Input: part model. Units: mm. Frame: model coordinates. A direction names the side the tool comes from. Coordinates: 2 decimals unless noted, no trailing zeros. Loops run counter-clockwise (first coordinate to the right, second up) from the corner with the lowest first, then second, coordinate; pieces in that order, holes last. Notation, with made-up numbers: (-36, 48.5) - (-13, 48.5) arc R24 cw to (-13, 85.5) - close; hole circle Ø2 at (-21, 56). An arc over 180 degrees is marked (long way). Use one line per item in the form item = value.
Autodesk Inventor part; units mm, degrees
ref_plane "YZ Plane" through (0, 0, 0) normal (1, 0, 0) x (0, 1, 0)
ref_plane "XZ Plane" through (0, 0, 0) normal (0, 1, 0) x (-1, 0, 0)
ref_plane "XY Plane" through (0, 0, 0) normal (0, 0, 1) x (1, 0, 0)
sketch "草图1" plane through (0, 0, 0) normal (0, 0, 1) x (1, 0, 0)
  line L0 (598.9577, 75) -> (600, -74.9964)
  line L1 (-601.0423, 75.1267) -> (600, -74.9964) construction
  line L2 (598.9577, 75) -> (-593.8092, -74.3553) construction
  line L3 (-300, 0) -> (-300, 100)
  line L4 (-300, -100) -> (600, -74.9964)
  line L5 (-300, 100) -> (598.9577, 75)
  line L6 (-300, 0) -> (-300, -100)
  line L7 (599.4789, 0) -> (-300, 0)
  line L8 (0, 0) -> (0, -189.9048)
  dimension "d0" = 150
  dimension "d31" = 75
  dimension "d32" = 0
  dimension "d33" = 100
  dimension "d34" = 100
  dimension "d35" = 100
  dimension "d51" = 300
extrude "拉伸1" add sketch "草图1" along normal mid plane 100
sketch "草图2" plane through (0, 0, 0) normal (0, 0, 1) x (1, 0, 0)
  circle A0 centre (-50, -120) radius 15
  line L0 (0, 0) -> (0, -405.8359)
  line L1 (0, 0) -> (-641.787, 0)
  line L2 (-80, -120) -> (-80, -93.888)
  line L3 (-300, -100) -> (600, -74.9964)
  line L4 (-20, -92.2211) -> (-20, -120)
  arc A1 (-80, -120) -> (-20, -120) centre (-50, -120) ccw
  dimension "d8" = 30
  dimension "d9" = 120
  dimension "d10" = 50
  dimension "d28" = 30
extrude "拉伸2" add sketch "草图2" along normal mid plane 100
fillet "圆角1" radius 30 1 edges at (-300, -100, 0)
sketch "草图4" plane through (0, 0, 50) normal (0, 0, 1) x (1, 0, 0)
  arc A0 (-300, -69.155) -> (-269.1669, -99.1434) centre (-270, -69.155) ccw
  circle A1 centre (-270, -69.155) radius 15
  point P0 (0, 0)
  dimension "d15" = 30
extrude "拉伸3" cut sketch "草图4" against normal blind 100
sketch "草图5" plane through (0, 0, 50) normal (0, 0, 1) x (1, 0, 0)
  arc A0 (-300, -69.155) -> (-269.1669, -99.1434) centre (-270, -69.155) ccw
  line L0 (-300, -69.155) -> (-300, 100)
  line L1 (598.9577, 75) -> (-300, 100)
  line L2 (-300, 100) -> (-300, -69.155)
  line L3 (-300, 100) -> (-300, 100)
  line L4 (-300, -69.155) -> (-295.2994, 99.8693)
  line L5 (-295.2994, 99.8693) -> (-300, 100)
  line L6 (598.9577, 75) -> (594.7823, -75.1413)
  line L7 (600, -74.9964) -> (-269.1669, -99.1434)
  line L8 (598.9577, 75) -> (600, -74.9964)
  line L9 (600, -74.9964) -> (598.9577, 75)
  point P0 (0, 0)
  point P1 (-603.2218, 0)
  point P2 (599.4789, 0)
  dimension "d20" = 90
extrude "拉伸4" cut sketch "草图5" against normal blind 100 contours L0 L1 L4 | L6 L8 L7
sketch "草图6" plane through (594.7823, -75.1413, 50) normal (0.9996135, -0.0277992, 0) x (0, 0, -1)
  line L0 (0, 0) -> (0, 150.1994)
  line L1 (0, 150.1994) -> (100, 150.1994)
  line L2 (50, 150.1994) -> (50, 0)
  line L3 (100, 0) -> (0, 0)
  line L4 (100, 150.1994) -> (100, 0)
  line L5 (15, 151) -> (85, 151)
  line L6 (85, 151) -> (85, 20)
  line L7 (85, 20) -> (15, 20)
  line L8 (15, 20) -> (15, 151)
  line L9 (15, 151) -> (85, 20) construction
  line L10 (85, 151) -> (15, 20) construction
  point P0 (50, 58.5778)
  point P1 (50, 85.5)
  point P2 (0, 100.4456)
  point P3 (0, 175.4618)
  point P4 (100, 175.4618)
  point P5 (100, 100.4456)
  dimension "d21" = 70
  dimension "d22" = 131
  dimension "d63" = 20
extrude "拉伸5" cut sketch "草图6" against normal through all contours L8 L5 L6 L1 | L1 L2 L7 L8 | L2 L1 L6 L7
sketch "草图7" plane through (0, 0, 0) normal (0, 0, 1) x (1, 0, 0)
  arc A0 (-300, -69.155) -> (-269.1669, -99.1434) centre (-270, -69.155) ccw
  circle A1 centre (-270, -69.155) radius 42.5
  point P0 (0, 0)
  dimension "d25" = 85
extrude "拉伸6" cut sketch "草图7" along normal mid plane 35
sketch "草图8" plane through (0, 0, 0) normal (0, 0, 1) x (1, 0, 0)
  line L0 (-632.149, 69.2216) -> (221.7891, 45.4736)
  line L1 (-295.2994, 99.8693) -> (-298.9189, -30.2798)
  line L2 (598.9577, 75) -> (-295.2994, 99.8693)
  circle A0 centre (-246.4307, 58.4948) radius 15
  arc A1 (-276.4191, 59.3288) -> (-216.4423, 57.6608) centre (-246.4307, 58.4948) ccw
  line L3 (-276.4191, 59.3288) -> (-275.3072, 99.3133)
  line L4 (-275.3072, 99.3133) -> (-520.3529, 106.128)
  line L5 (-275.3127, 99.114) -> (-215.3359, 97.446)
  line L6 (598.9522, 74.8007) -> (-295.305, 99.67)
  line L7 (-215.3359, 97.446) -> (-216.4423, 57.6608)
  point P0 (0, 0)
  dimension "d36" = 40
  dimension "d37" = 30
  dimension "d38" = 60
  dimension "d39" = 50
  dimension "d40" = 90
  dimension "d41" = 60
extrude "拉伸7" add sketch "草图8" along normal mid plane 70 contours L3 L5 L7 L0 A0 | L0 A0 A1 | A0 L0 | L0 A0
sketch "草图9" plane through (0, 0, 50) normal (0, 0, 1) x (1, 0, 0)
  arc A0 (-276.4191, 59.3288) -> (-216.4423, 57.6608) centre (-246.4307, 58.4948) ccw
  circle A1 centre (-246.4307, 58.4948) radius 15
  point P0 (0, 0)
  dimension "d44" = 30
extrude "拉伸8" cut sketch "草图9" against normal through all
sketch "草图10" plane through (-276.4191, 59.3288, -35) normal (-0.9996135, 0.0277992, 0) x (0, 0, 1)
  line L0 (0, 39.8006) -> (70, 39.8006)
  line L1 (35, 39.8006) -> (35, -30)
  line L2 (0, -30) -> (70, -30)
  line L3 (17.5, 39.8006) -> (52.5, 39.8006)
  line L4 (52.5, 39.8006) -> (52.5, -30)
  line L5 (52.5, -30) -> (17.5, -30)
  line L6 (17.5, -30) -> (17.5, 39.8006)
  line L7 (17.5, 39.8006) -> (52.5, -30) construction
  line L8 (52.5, 39.8006) -> (17.5, -30) construction
  point P0 (35, -51.6216)
  point P1 (35, 4.9003)
  dimension "d47" = 35
extrude "拉伸9" cut sketch "草图10" against normal blind 60
sketch "草图13" plane through (-295.2994, 99.8693, 50) normal (0.0277992, 0.9996135, 0) x (0.9996135, -0.0277992, 0)
  line L0 (0, 15) -> (0, 85)
  line L1 (0, 50) -> (323.6348, 50)
  line L2 (0, 100) -> (31.6549, 100)
  line L3 (200, 0) -> (0, 0)
  line L4 (0, 0) -> (0, 100)
  line L5 (0, 100) -> (200, 100)
  line L6 (200, 100) -> (200, 0)
  line L7 (200, 0) -> (0, 100) construction
  line L8 (0, 0) -> (200, 100) construction
  line L9 (894.6029, 100) -> (894.6029, 0)
  line L10 (844.6029, 100) -> (894.6029, 100)
  line L11 (894.6029, 100) -> (894.6029, 0)
  line L12 (894.6029, 0) -> (844.6029, 0)
  line L13 (844.6029, 0) -> (844.6029, 100)
  line L14 (844.6029, 100) -> (894.6029, 0) construction
  line L15 (894.6029, 100) -> (844.6029, 0) construction
  point P0 (297.9616, 50)
  point P1 (100, 50)
  point P2 (869.6029, 50)
  dimension "d64" = 200
  dimension "d65" = 50
extrude "拉伸12" add sketch "草图13" along normal blind 10
properties part number "DipperParent" material "钢，高强度，低合金"
Q1. First-contact query: P1, Ø6, axis at x = 469, z = -4.5, coming from the -Y side; P2, Ø14, axis at y = -102, z = 11, coming from the +X side; P3, Ø6, axis at x = 386.5, z = -8.5, coming from the -Y side. Flat tips, straight axial feed; report the tip coordinate or a pass-through.
Check values:
P1 = -78.72
P2 = -20
P3 = -81.01
Q2. Cut plane D-D, the plane x = -171. Return loops of the section in (y, z).
Check values:
outline = (-96.42, -50) - (106.42, -50) - (106.42, 50) - (-96.42, 50) - close; hole (-33.84, -35) - (96.41, -35) - (96.41, 35) - (-33.84, 35) - close
Q3. Cut plane B-B, the plane z = 6.5. Return loops of the section in (x, y) (3 decimals), then the cut area to 3 significant figures.
Check values:
outline = (-299.14, -38.217) arc R42.5 cw to (-287.855, -30.587) - (-298.919, -30.28) - close; (-295.299, 99.869) - (-95.377, 94.309) - (-95.099, 104.306) - (-295.021, 109.865) - close; (-250.029, -31.639) arc R42.5 cw to (-239.074, -98.307) - (-80, -93.888) - (-80, -120) arc R30 ccw to (-20, -120) - (-20, -92.221) - (594.782, -75.141) - (595.338, -55.149) - close; (548.977, 76.39) - (598.958, 75) - (599.236, 84.996) - (549.255, 86.386) - close; hole circle Ø30 at (-50, -120)
area = 40,500 mm²
Q4. Cut plane A-A, the plane x = -50. Return loops of the section in (y, z).
Check values:
outline = (-150, -50) - (-135, -50) - (-135, 50) - (-150, 50) - close; (-105, -50) - (93.05, -50) - (93.05, -35) - (-37.2, -35) - (-37.2, 35) - (93.05, 35) - (93.05, 50) - (-105, 50) - close
Q5. Pull-direction query (Z, two-part tool) for faces 4 (the cylindrical face through (-246.605, 28.495, -26.373)), 5 (the flat face through (156, 21, 35)), 6 (the cylindrical face through (-232.123, 63, -33.523)); classes: pulls with the +Z half, pulls with the -Z half, needs draft (parallel to the pull), parting line crosses it, or undercut.
Check values:
face_4 = undercut
face_5 = undercut
face_6 = needs draft
Q6. Cut plane C-C, the plane y = -16.5. Return loops of the section in (x, z).
Check values:
outline = (-298.54, -50) - (596.41, -50) - (596.41, -35) - (-298.54, -35) - close; (-298.54, 35) - (596.41, 35) - (596.41, 50) - (-298.54, 50) - close
Q7. Set-up query: faces 1 (the cylindrical face through (-232.123, 63, 33.978)), 2 (the cylindrical face through (-246.605, 28.495, 26.127)), 3 (the flat face through (-20, -106, -1)). Return all of +Z, -Z, +X, -X, +Y, -Y with unobstructed straight access to the full face (end or side cutting, diameter ignored); none if empty.
Check values:
face_1 = +Z, -Z
face_2 = none
face_3 = +Z, -Z, +X, -Y
Q8. Ray query, line 1 along Z through (x, y) = (59, 71); line 2 along Y through (x, z) = (-270, 25) (3 decimals); line 3 along X through (y, z) = (-118.5, -4). Return the intervals inside material, ascending. Write a range as [from, to].
Check values:
line_1 = [-50, -35], [35, 50]
line_2 = [-99.155, -84.155], [-54.155, -31.084], [39.934, 98.966], [99.166, 109.17]
line_3 = [-80, -64.92], [-35.08, -20]
